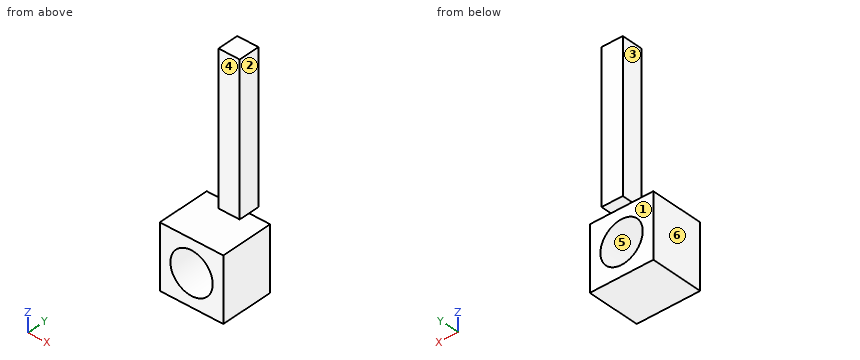
from build123d import *

# Parameters (mm, degrees)
F0_W     = 30
F0_H     = 30
F1_DEPTH = 25
F2_R     = 10
F3_DEPTH = 25
F4_W     = 10
F4_H     = 10
F5_DEPTH = 70


with BuildPart() as f1:
    # F0 (on Front) → F1 (new body)
    with BuildSketch(Plane.XZ):
        Rectangle(F0_W, F0_H)
    extrude(amount=F1_DEPTH)

    # F2 (on face) → F3 (cut)
    with BuildSketch(Plane.XZ.offset(25)):
        Circle(F2_R)
    extrude(amount=-F3_DEPTH, mode=Mode.SUBTRACT)

    # F4 (on face) → F5 (join)
    with BuildSketch(Plane.XY.offset(15)):
        Rectangle(F4_W, F4_H)
    extrude(amount=F5_DEPTH)


solid = f1.part
Source: CAD feature listing. Evaluate the final solid. Frame: model axes, mm. Face numbers are marked on the shaded views. A direction names the side the tool comes from. Coordinates: 2 decimals unless noted, no trailing zeros. Loops run counter-clockwise (first coordinate to the right, second up) from the corner with the lowest first, then second, coordinate; pieces in that order, holes last. Notation, with made-up numbers: (5, 56) - (49, 56) arc R13 cw to (49, 78) - close; hole circle Ø8 at (51.5, -25.75). An arc over 180 degrees is marked (long way). One line per item, written item: value. Start each with the question number.
1. Section A-A (z = 0). Return the cut outline in (x, y), and give its area (3 significant figures).
2. Contact query for flat-ended pins moving along their axis: P1, Ø8, axis at y = -1, z = 52.5, coming from the -X side; P2, Ø8, axis at x = 2, z = 46, coming from the -Y side; P3, Ø12, axis at y = -9.5, z = 25, coming from the +X side. Output: stop coordinate, or through.
3. Section D-D (x = 12). Return the cut outline in (y, z).
4. Mould query, pull axis X, two halves, no side actions, for the marked faces 4, 5 and 6. Classes: pulls with the +X half, pulls with the -X half, needs draft (parallel to the pull), parting line crosses it, or undercut.
5. Ray query, L1, parallel to Z at x = 0, y = -18; L2, parallel to X at y = -2.5, z = 19.5. Return the intervals inside material, ascending.
6. Set-up query: the marked faces 1, 2 and 3. Return all of +Z, -Z, +X, -X, +Y, -Y with unobstructed straight access to the full face (end or side cutting, diameter ignored); none if empty.
7. Section C-C (y = 2.5). Return the cut outline in (x, z), and give its area (3 significant figures).
8. Section B-B (x = 0). Return the cut outline in (y, z).
Verdict:
1. outline: (-15, -25) - (-10, -25) - (-10, 0) - (-15, 0) - close; (10, -25) - (15, -25) - (15, 0) - (10, 0) - close
1. area: 250 mm2
2. P1: stops at x = -5
2. P2: stops at y = -5
2. P3: stops at x = 5
3. outline: (-25, -15) - (0, -15) - (0, 15) - (-25, 15) - close
4. face 4: needs draft
4. face 5: undercut
4. face 6: pulls with the -X half
5. L1: z = -15 to -10, 10 to 15
5. L2: x = -5 to 5
6. face 1: -Z, +X, -X, +Y
6. face 2: +Z, +X, +Y, -Y
6. face 3: +Z, -X, +Y, -Y
7. outline: (-5, 15) - (5, 15) - (5, 85) - (-5, 85) - close
7. area: 700 mm2
8. outline: (-25, -15) - (0, -15) - (0, -10) - (-25, -10) - close; (-25, 10) - (0, 10) - (0, 15) - (5, 15) - (5, 85) - (-5, 85) - (-5, 15) - (-25, 15) - close
